Part model, mm, in its own coordinate system. A direction names the side the tool comes from. Give positions to 0.01 mm unless a question says otherwise; leave off trailing zeros. Write each loop counter-clockwise with the first axis right and the second up, starting at its lowest first coordinate (ties: lowest second). Pieces come first, ordered by that corner, then holes.
from build123d import *

# Parameters (mm, degrees)
SKETCH1_R                = 12.55
SKETCH1_R_2              = 1.925
BOSS_EXTRUDE1_DEPTH      = 10
FILLET1_R                = 5
BOSS_EXTRUDE2_DEPTH      = 5
BOSS_EXTRUDE2_DEPTH_BACK = 15
SKETCH2_R                = 1.925
SKETCH3_R                = 1.925
BOSS_EXTRUDE3_DEPTH      = 2
BOSS_EXTRUDE4_START      = -20
BOSS_EXTRUDE4_OUTLINE_R  = 1.925
BOSS_EXTRUDE4_DEPTH      = 2
SKETCH4_W                = 12.5
SKETCH4_H                = 20
BOSS_EXTRUDE5_DEPTH      = 1.7
SKETCH5_W                = 1.7
SKETCH5_H                = 10
BOSS_EXTRUDE6_DEPTH      = 14


# Read off the part's stored shape, not the designer's step: Boss-Extrude4
with BuildPart() as part:
    # Sketch1 → Boss-Extrude1 (new body)
    with BuildSketch(Plane(origin=(0, 0, 0), x_dir=(1, 0, 0), z_dir=(0, 1, 0))):
        with Locations(Location((0, 0, 0), (0, 0, 270))):
            Circle(SKETCH1_R)
        with Locations(Location((0, 0, 0), (0, 0, 270))):
            Circle(SKETCH1_R_2, mode=Mode.SUBTRACT)
    extrude(amount=BOSS_EXTRUDE1_DEPTH)

    # Fillet1
    fillet1_edges = [part.edges().sort_by_distance(p)[0] for p in [
        (0, 0, -12.55),
        (0, 10, -12.55),
    ]]
    fillet(fillet1_edges, radius=FILLET1_R - 0.0001)  # a hair under: the kernel refuses the full size

    # Sketch2 → Boss-Extrude2 (add, two sides: drawn at the far end of the back side and taken through both)
    with BuildSketch(Plane.XZ.offset(-BOSS_EXTRUDE2_DEPTH_BACK)):
        with Locations(Location((0, 0, 0), (0, 0, 270))):
            Circle(SKETCH2_R)
    extrude(amount=BOSS_EXTRUDE2_DEPTH + BOSS_EXTRUDE2_DEPTH_BACK)

    # Sketch3 → Boss-Extrude3 (add)
    with BuildSketch(Plane.XZ.offset(5)):
        with BuildLine():
            Line((20, 5), (20, 17.5))
            ThreePointArc((20, 17.5), (5.770309443, 14.004874621), (-3.696538076, 2.821011566))
            ThreePointArc((-3.696538076, 2.821011566), (-1.488891861, -4.405190237), (4.65, 0))
            ThreePointArc((4.65, 0), (11.70086168, 4.416104641), (20, 5))
        make_face()
        with Locations(Location((0, 0, 0), (0, 0, 270))):
            Circle(SKETCH3_R, mode=Mode.SUBTRACT)
    extrude(amount=-BOSS_EXTRUDE3_DEPTH)

    # Boss-Extrude4 outline → Boss-Extrude4 (add)
    with BuildSketch(Plane.XZ.offset(5).offset(BOSS_EXTRUDE4_START)):
        with BuildLine():
            ThreePointArc((-3.696538076, 2.821011566), (-1.488891861, -4.405190237), (4.65, 0))
            ThreePointArc((4.65, 0), (11.70086168, 4.416104641), (20, 5))
            Line((20, 5), (20, 17.5))
            ThreePointArc((20, 17.5), (5.770309443, 14.004874621), (-3.696538076, 2.821011566))
        make_face()
        Circle(BOSS_EXTRUDE4_OUTLINE_R, mode=Mode.SUBTRACT)
    extrude(amount=BOSS_EXTRUDE4_DEPTH)

    # Sketch4 → Boss-Extrude5 (add)
    with BuildSketch(Plane(origin=(20, 0, 0), x_dir=(0, 0, -1), z_dir=(1, 0, 0))):
        with Locations((-11.25, 5)):
            Rectangle(SKETCH4_W, SKETCH4_H)
    extrude(amount=-BOSS_EXTRUDE5_DEPTH)

    # Sketch5 → Boss-Extrude6 (add)
    with BuildSketch(Plane(origin=(0, 0, 5), x_dir=(-1, 0, 0), z_dir=(0, 0, -1))):
        with BuildLine():
            ThreePointArc((-25.307916987, 9.896233666), (-21.967917982, 8.39623271), (-20.6, 5))
            Line((-20.6, 5), (-20, 5))
            Line((-20, 5), (-20, 15))
            ThreePointArc((-20, 15), (-21.62390923, 11.376865599), (-25.307916987, 9.896233666))
        make_face()
        with BuildLine():
            Line((-20, 5), (-20.6, 5))
            ThreePointArc((-20.6, 5), (-21.967917982, 1.60376729), (-25.307916987, 0.103766334))
            ThreePointArc((-25.307916987, 0.103766334), (-21.62390923, -1.376865599), (-20, -5))
            Line((-20, -5), (-20, 5))
        make_face()
        with BuildLine():
            ThreePointArc((-25.307916987, 0.103766334), (-21.967917982, 1.60376729), (-20.6, 5))
            Line((-20.6, 5), (-22.6, 5))
            ThreePointArc((-22.6, 5), (-25.5, 2.1), (-28.4, 5))
            Line((-28.4, 5), (-30.4, 5))
            ThreePointArc((-30.4, 5), (-28.964823228, 1.535176772), (-25.5, 0.1))
            ThreePointArc((-25.5, 0.1), (-25.403975548, 0.102752972), (-25.307916987, 0.103766334))
        make_face()
        with BuildLine():
            Line((-22.6, 5), (-20.6, 5))
            ThreePointArc((-20.6, 5), (-21.967917982, 8.39623271), (-25.307916987, 9.896233666))
            ThreePointArc((-25.307916987, 9.896233666), (-25.403975548, 9.897247028), (-25.5, 9.9))
            ThreePointArc((-25.5, 9.9), (-28.964823228, 8.464823228), (-30.4, 5))
            Line((-30.4, 5), (-28.4, 5))
            ThreePointArc((-28.4, 5), (-25.5, 7.9), (-22.6, 5))
        make_face()
        with Locations((-19.15, 0)):
            Rectangle(SKETCH5_W, SKETCH5_H)
        with Locations((-19.15, 10)):
            Rectangle(SKETCH5_W, SKETCH5_H)
    extrude(amount=-BOSS_EXTRUDE6_DEPTH)


solid = part.part
1) 3-axis set-ups, long thin cutter, end or side, ignore diameter. For faces 4 (the cylindrical face through (10.79, -4.01, 4.09)), 5 (the cylindrical face through (-1.605, -4.014, -4.364)), 6 (the cylindrical face through (-1.17, -1.48, 1.53)): which of +Z, -Z, +X, -X, +Y, -Y reach the whole face in a straight line?
Check result:
face 4: -Z, -Y
face 5: -Y
face 6: none
2) Mould opens along Y. For faces 1 (the flat face through (22, 5, 19)), 2 (the flat face through (8, 15, 7)), 3 (the flat face through (-2, 10, 2)) say: +Y half, -Y half, draft (parallel to the pull), parting line (faces both ways), or undercut.
Check result:
face 1: draft
face 2: +Y half
face 3: undercut
3) Saw through at A-A (y = 5.5). Write the cut outline in (x, z).
Check result:
outline: circle Ø25.05 at (0, 0); (18.3, 5) - (22.64, 5) - (22.64, 19) - (18.3, 19) - close; (28.36, 5) - (30.37, 5) - (30.37, 19) - (28.36, 19) - close
4) Saw through at D-D (z = -3.5). State how many separate pieces and enclosed holes the cut face has, and give its area (3 significant figures).
Check result:
separate pieces: 3
enclosed holes: 0
area: 243 mm2
5) Flat gauge pins, fed straight in: P1, Ø4, axis at x = 20.5, y = 1, coming from the -Z side; P2, Ø1, axis at x = -3, y = 9.5, coming from the +Z side; P3, Ø6, axis at x = 18.5, z = -1, coming from the -Y side; P4, Ø5, axis at y = 0.5, z = -3, coming from the +X side. Where does each tip first touch, or does it go through?
Check result:
P1: stops at z = 5
P2: stops at z = 10.13
P3: passes through
P4: stops at x = 11.87
6) Saw through at B-B (y = 9). Write the cut outline in (x, z).
Check result:
outline: circle Ø21.1 at (0, 0); (18.3, 5) - (28.33, 5) - (28.33, 19) - (18.3, 19) - close
7) Drill centre lines: L1, parallel to Y at x = 25.5, z = 9.25; L2, parallel to Y at x = 6, z = -4.5; L3, parallel to X at y = 1.75, z = 5.5. Where is each one in solid material? Low to high.
Check result:
L1: y = 0.1 to 2.1, 7.9 to 9.9
L2: y = 0 to 10
L3: x = -9.93 to 9.93, 18.3 to 29.17
